Autodesk Inventor part; units mm, degrees
ref_plane "YZ Plane" through (0, 0, 0) normal (1, 0, 0) x (0, 1, 0)
ref_plane "XZ Plane" through (0, 0, 0) normal (0, 1, 0) x (-1, 0, 0)
ref_plane "XY Plane" through (0, 0, 0) normal (0, 0, 1) x (1, 0, 0)
sketch "Sketch1" plane through (0, 0, 0) normal (0, 0, 1) x (1, 0, 0)
  line L0 (0, 0) -> (25.4, 0)
  line L1 (25.4, 0) -> (25.4, 25.4)
  line L2 (25.4, 25.4) -> (0, 25.4)
  line L3 (0, 25.4) -> (0, 0)
  line L4 (1.5875, 23.8125) -> (23.8125, 23.8125)
  line L5 (23.8125, 23.8125) -> (23.8125, 1.5875)
  line L6 (23.8125, 1.5875) -> (1.5875, 1.5875)
  line L7 (1.5875, 1.5875) -> (1.5875, 23.8125)
  dimension "d0" = 25.4
  dimension "d1" = 25.4
  dimension "d2" = 1.5875
extrude "Extrusion1" add sketch "Sketch1" against normal blind 127
sketch "Sketch2" plane through (0, 0, 0) normal (0, -1, 0) x (1, 0, 0)
  line L0 (0, -127) -> (25.4, -127)
  line L1 (0, 0) -> (25.4, 0)
  point P0 (12.7, -12.7)
  point P1 (12.7, -114.3)
  point P2 (12.7, -88.9)
  point P3 (12.7, -63.5)
  point P4 (12.7, -127)
  dimension "d5" = 25.4
  dimension "d6" = 25.4
  dimension "d7" = 12.7
  dimension "d8" = 12.7
hole "Hole1" at (12.7, 0, -12.7) at (12.7, 0, -114.3) at (12.7, 0, -88.9) at (12.7, 0, -63.5) direction (0, 1, 0) diameter 6.35 depth 25.4 tip angle 118
sketch "Sketch3" plane through (0, 0, 0) normal (-1, 0, 0) x (0, 0, 1)
  line L0 (-127, 25.4) -> (-127, 0)
  point P0 (-114.3, 12.7)
  point P1 (-76.2, 12.7)
  dimension "d25" = 12.7
  dimension "d27" = 38.1
hole "Hole2" at (0, 12.7, -114.3) at (0, 12.7, -76.2) direction (1, 0, 0) diameter 6.35 depth 25.4 tip angle 118
properties part number "1tube_6"
Source: CAD feature listing. Evaluate the final solid. Frame: model axes, mm. A direction names the side the tool comes from. Coordinates: 2 decimals unless noted, no trailing zeros. Write each loop counter-clockwise with the first axis right and the second up, starting at its lowest first coordinate (ties: lowest second). Pieces come first, ordered by that corner, then holes. Notation, with made-up numbers: (77, -33.5) -> (119, -33.5) arc R14 cw to (119, -22.5) -> close; hole circle Ø3 at (8, -33.5). An arc over 180 degrees is marked (long way). Return JSON: item names as keys, results as strings. Group by question number.
1) Section query D-D, the plane z = -114.3. Return loops of the section in (x, y) (1 decimal).
2) Set-up query: faces 4 (the face through (23.812, 13, -63)), 5 (the face through (14.63, 0.8, -86.38)). Return all of +Z, -Z, +X, -X, +Y, -Y with unobstructed straight access to the full face (end or side cutting, diameter ignored); none if empty.
3) Section query A-A, the plane y = 17.75. Return loops of the section in (x, z).
4) Ray query, line 1 along Z through (x, y) = (12.7, 0.8) (3 decimals); line 2 along Z through (x, y) = (24.8, 12.7) (3 decimals); line 3 along Y through (x, z) = (22, -103). Return the intervals inside material, ascending.
5) Section query B-B, the plane z = -63.5. Return loops of the section in (x, y) (1 decimal).
6) Mould query, pull axis Y, two halves, no side actions, for faces 1 (the face through (18, 1.588, -63)), 2 (the face through (18, 0, -63)), 3 (the face through (1, 13, 0)). Classes: +Y half, -Y half, draft (parallel to the pull), parting line (faces both ways), or undercut.
From the geometry:
{
 "1": {"outline": "(0, 0) -> (9.5, 0) -> (9.5, 1.6) -> (1.6, 1.6) -> (1.6, 9.5) -> (0, 9.5) -> close; (0, 15.9) -> (1.6, 15.9) -> (1.6, 23.8) -> (9.5, 23.8) -> (9.5, 25.4) -> (0, 25.4) -> close; (15.9, 0) -> (25.4, 0) -> (25.4, 9.5) -> (23.8, 9.5) -> (23.8, 1.6) -> (15.9, 1.6) -> close; (15.9, 23.8) -> (23.8, 23.8) -> (23.8, 15.9) -> (25.4, 15.9) -> (25.4, 25.4) -> (15.9, 25.4) -> close"},
 "2": {"face 4": "+Z, -Z", "face 5": "+Y, -Y"},
 "3": {"outline": "(0, -127) -> (1.59, -127) -> (1.59, 0) -> (0, 0) -> close; (23.81, -127) -> (25.4, -127) -> (25.4, 0) -> (23.81, 0) -> close"},
 "4": {"line 1": "-127 to -117.475, -111.125 to -92.075, -85.725 to -66.675, -60.325 to -15.875, -9.525 to 0", "line 2": "-127 to -117.475, -111.125 to -79.375, -73.025 to 0", "line 3": "0 to 1.59, 23.81 to 25.4"},
 "5": {"outline": "(0, 0) -> (9.5, 0) -> (9.5, 1.6) -> (1.6, 1.6) -> (1.6, 23.8) -> (9.5, 23.8) -> (9.5, 25.4) -> (0, 25.4) -> close; (15.9, 0) -> (25.4, 0) -> (25.4, 25.4) -> (15.9, 25.4) -> (15.9, 23.8) -> (23.8, 23.8) -> (23.8, 1.6) -> (15.9, 1.6) -> close"},
 "6": {"face 1": "undercut", "face 2": "-Y half", "face 3": "draft"}
}
